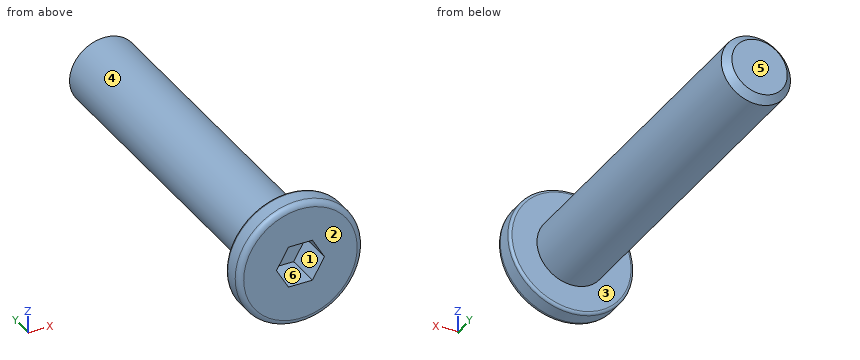
Autodesk Inventor part; units mm, degrees
ref_plane "YZ Plane" through (0, 0, 0) normal (1, 0, 0) x (0, 1, 0)
ref_plane "XZ Plane" through (0, 0, 0) normal (0, 1, 0) x (-1, 0, 0)
ref_plane "XY Plane" through (0, 0, 0) normal (0, 0, 1) x (1, 0, 0)
sketch "Boceto1" plane through (0, 0, 0) normal (0, 1, 0) x (-1, 0, 0)
  circle A0 centre (0, 0) radius 4.5
  dimension "d0" = 9
extrude "Extrusión1" add sketch "Boceto1" along normal blind 1.6
sketch "Boceto2" plane through (0, 1.6, 0) normal (0, 1, 0) x (1, 0, 0)
  circle A0 centre (0, 0) radius 2.5
  dimension "d3" = 5
extrude "Extrusión2" add sketch "Boceto2" along normal blind 25
fillet "Empalme1" radius 0.4 1 edges at (4.5, 0, 0)
fillet "Empalme2" radius 0.2 1 edges at (4.5, 1.6, 0)
sketch "Boceto3" plane through (0, 0, 0) normal (0, -1, 0) x (1, 0, 0)
  line L0 (-1.7321, 0) -> (-0.866, 1.5)
  line L1 (-0.866, 1.5) -> (0.866, 1.5)
  line L2 (0.866, 1.5) -> (1.7321, 0)
  line L3 (1.7321, 0) -> (0.866, -1.5)
  line L4 (0.866, -1.5) -> (-0.866, -1.5)
  line L5 (-0.866, -1.5) -> (-1.7321, 0)
  point P0 (0, 0)
  point P1 (0, 0)
  dimension "d8" = 3
extrude "Extrusión3" cut sketch "Boceto3" against normal blind 2.5
chamfer "Chaflán1" distance 0.5 angle 45 1 edges at (-2.5, 26.6, 0)
thread "Rosca2"
properties part number "Perno M5x8 cabeza plana" material "Hierro, gris"
Input: part model. Units: mm. Frame: model coordinates. Face numbers are marked on the shaded views. A direction names the side the tool comes from. Give positions to 0.01 mm unless a question says otherwise; leave off trailing zeros. Loops run counter-clockwise (first coordinate to the right, second up) from the corner with the lowest first, then second, coordinate; pieces in that order, holes last. Notation, with made-up numbers: (-32, 74.5) - (1, 74.5) arc R20 cw to (1, 106.5) - close; hole circle Ø2 at (72.5, -4.75). An arc over 180 degrees is marked (long way). Use CSV: the item, a comma, the result in double quotes. Start each with the question number.
Item 1: Line query: line 1 (Y direction, x = 0.5, z = 3.25); line 2 (Y direction, x = -0.5, z = 0.25); line 3 (Z direction, x = 2, y = 11.5). Output: solid intervals per line, ascending.
Item 2: Contact query for flat-ended pins moving along their axis: P1, Ø5, axis at x = 1.5, y = 9, coming from the -Z side; P2, Ø0.5, axis at x = 0.5, y = 1.5, coming from the +Z side; P3, Ø5, axis at y = 3.5, z = 3, coming from the -X side. Output: stop coordinate, or through.
Item 3: Reachability of the marked faces 1, 2 and 3 from +Z, -Z, +X, -X, +Y, -Y: full face, straight path, thin tool, end or side. Return the list, or none.
Item 4: Section A-A on x = 0. Return loops of the section in (y, z), then the cut area to 3 significant figures.
Item 5: Mould query, pull axis Z, two halves, no side actions, for the marked faces 4, 5 and 6. Classes: pulls with the +Z half, pulls with the -Z half, needs draft (parallel to the pull), parting line crosses it, or undercut.
Item 6: Section B-B on y = 15.75. Return loops of the section in (x, z), then the cut area to 3 significant figures.
Ans:
1,line 1,"y = 0 to 1.6"
1,line 2,"y = 2.5 to 26.6"
1,line 3,"z = -1.5 to 1.5"
2,P1,"stops at z = -2.5"
2,P2,"stops at z = 4.49"
2,P3,"stops at x = -4.22"
3,face 1,"-Y"
3,face 2,"+Z, -Z, +X, -X, -Y"
3,face 3,"+Y"
4,outline,"(0, -4.1) arc R0.4 ccw to (0.4, -4.5) - (1.4, -4.5) arc R0.2 ccw to (1.6, -4.3) - (1.6, -2.5) - (26.1, -2.5) - (26.6, -2) - (26.6, 2) - (26.1, 2.5) - (1.6, 2.5) - (1.6, 4.3) arc R0.2 ccw to (1.4, 4.5) - (0.4, 4.5) arc R0.4 ccw to (0, 4.1) - (0, 1.5) - (2.5, 1.5) - (2.5, -1.5) - (0, -1.5) - close"
4,area,"132 mm2"
5,face 4,"parting line crosses it"
5,face 5,"needs draft"
5,face 6,"undercut"
6,outline,"circle Ø5 at (0, 0)"
6,area,"19.6 mm2"
